The drawing under review shows one solid part. Ordinate dimensions are in mm from its lowest x, y, z. Give positions to 0.01 mm unless a question says otherwise; leave off trailing zeros. Order: outer loops, then holes, each group sorted by start corner. A loop starts at its lowest first (then second) coordinate and runs counter-clockwise, first axis right, second up. Notation, with made-up numbers: (14.5, 41.25) - (39.5, 41.25) arc R24 cw to (39.5, 80.25) - close; hole circle Ø10 at (39.5, 32). An arc over 180 degrees is marked (long way). Use CSV: the item, a comma, the result in double quotes. Start each with the question number.
1. Take a section at C-C, the plane z = 177. State the section outline as (x, y) points.
2. Take a section at A-A, the plane x = 10. State the section outline as (y, z) points.
3. For pin 1 (8 mm diameter, centred on x = 5, z = 192, fed in from +Y); pin 2 (12 mm diameter, centred on x = 11, z = 156, fed in from -Y); pin 3 (8 mm diameter, centred on y = 17, z = 148, fed in from +X), all flat-tipped, find the tip position at first contact; note any pin that passes through.
4. To check wall thickness, follow line 1 (Z direction, x = 6, y = 16); line 2 (Y direction, x = 10.5, z = 296); line 3 (Y direction, x = 11.25, z = 155.5). State the ranges of each line that lie inside material, in increasing order. Write a range as [from, to].
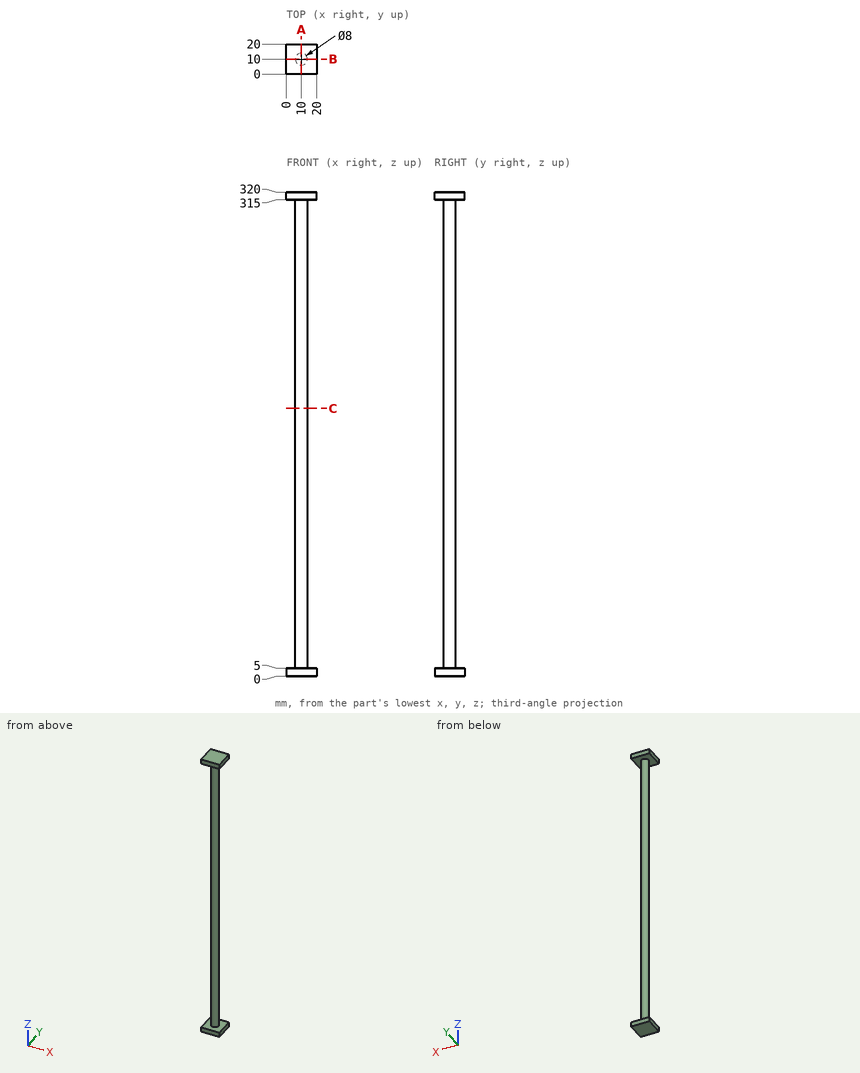
Determined:
1,outline,"circle Ø8 at (10, 10)"
2,outline,"(0, 0) - (20, 0) - (20, 5) - (14, 5) - (14, 315) - (20, 315) - (20, 320) - (0, 320) - (0, 315) - (6, 315) - (6, 5) - (0, 5) - close"
3,pin 1,"stops at y = 13.87"
3,pin 2,"stops at y = 6"
3,pin 3,"stops at x = 12.65"
4,line 1,"z = [0, 5], [315, 320]"
4,line 2,"y = [6.03, 13.97]"
4,line 3,"y = [6.2, 13.8]"
